Read the model definition and answer for the solid it produces. Units are mm, in the model's axes. Coordinates: 2 decimals unless noted, no trailing zeros. Loops run counter-clockwise (first coordinate to the right, second up) from the corner with the lowest first, then second, coordinate; pieces in that order, holes last. Notation, with made-up numbers: (-3, 17.25) -> (24, 17.25) arc R32 cw to (24, 54.25) -> close; hole circle Ø3 at (51.5, 73). An arc over 180 degrees is marked (long way). Answer as a JSON object with one key per item and string values. Group by question number.
1) Section A-A, the plane z = 4.75 is taken. Give the vertices of the cut face in (x, y).
2) Section C-C, the plane x = 285.5 is taken. Give the vertices of the cut face in (y, z).
3) Flat-ended cylindrical pins translate along their axes: P1, Ø1.2, axis at x = 115.5, z = 1.5, coming from the +Y side; P2, Ø0.9, axis at x = 151, y = 271, coming from the -Z side; P3, Ø5, axis at y = 147.5, z = 5, coming from the +X side. Find the tip coordinate at first contact, or state that the pin passes through.
4) Consider probe 1 along X at (y, z) = (142, 1.5); probe 2 along Y at (x, z) = (70, 9.25); probe 3 along X at (y, z) = (68.5, 8.5). Determine where each line is inside the solid, lowest interval first. Write a range as [from, to].
5) Section B-B, the plane y = 170 is taken. Give the vertices of the cut face in (x, z).
from build123d import *

# Parameters (mm, degrees)
EXTRUDE_1_DEPTH     = 10
CUT_EXTRUDE_1_DEPTH = 431.232495286


with BuildPart() as part:
    # 草圖1 → 填料-伸長1 (new body)
    with BuildSketch(Plane.XY):
        Polygon((250, 76.558764576), (304.147622093, 51.309313723), (304.147622093, 0), (154.147622093, 0), (0, 0), (0, 350), (250, 350), align=None)
    extrude(amount=EXTRUDE_1_DEPTH)

    # 草圖3 → 除料-伸長1 (cut, through all)
    with BuildSketch(Plane(origin=(250, 0, 0), x_dir=(0, 0, -1), z_dir=(1, 0, 0))):
        Polygon((0, 350), (-10, 350), (-10, 270), (-7.5, 270), (-7.5, 273), (-2.5, 273), (-2.5, 270), (0, 270), align=None)
    extrude(amount=-CUT_EXTRUDE_1_DEPTH, mode=Mode.SUBTRACT)


solid = part.part
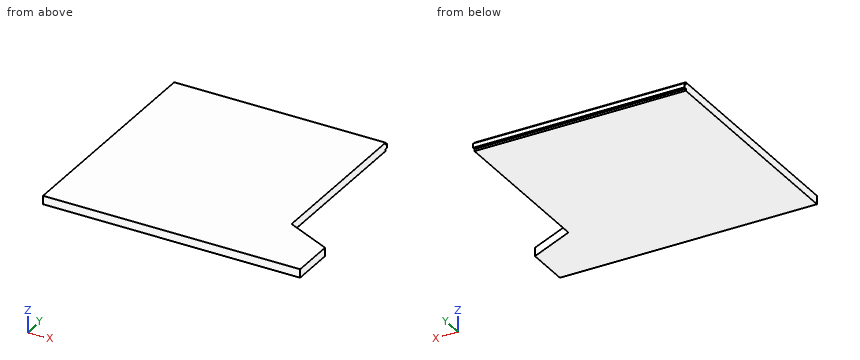
Determined:
{
 "1": {"outline": "(0, 0) -> (304.15, 0) -> (304.15, 51.31) -> (250, 76.56) -> (250, 273) -> (0, 273) -> close"},
 "2": {"outline": "(0, 0) -> (60, 0) -> (60, 10) -> (0, 10) -> close"},
 "3": {"P1": "y = 270", "P2": "z = 2.5", "P3": "x = 250"},
 "4": {"probe 1": "[0, 250]", "probe 2": "[0, 270]", "probe 3": "[0, 267.28]"},
 "5": {"outline": "(0, 0) -> (250, 0) -> (250, 10) -> (0, 10) -> close"}
}
